Geometry check sheet. Reference: the model listing, model coordinates, mm. Face numbers are marked on the shaded views. A direction names the side the tool comes from. Coordinates: 2 decimals unless noted, no trailing zeros. Loops run counter-clockwise (first coordinate to the right, second up) from the corner with the lowest first, then second, coordinate; pieces in that order, holes last. Notation, with made-up numbers: (58, 70) -> (76, 70) arc R18 ccw to (76, 88) -> close; hole circle Ø11 at (66, -4.5). An arc over 180 degrees is marked (long way). Answer as a JSON object with one key per item and string values.
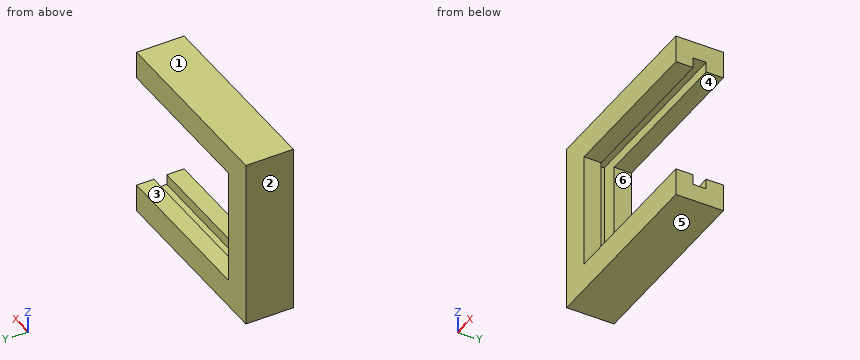
from build123d import *

# Parameters (mm, degrees)
SKETCH1_W           = 19.8
SKETCH1_H           = 5.5
SKETCH1_W_2         = 15.8
SKETCH1_H_2         = 1.5
BOSS_EXTRUDE1_DEPTH = 20.5
SKETCH2_W           = 18.5
SKETCH2_H           = 13.4
CUT_EXTRUDE1_DEPTH  = 6.5
SKETCH3_W           = 19.8
SKETCH3_H           = 5.5
BOSS_EXTRUDE2_DEPTH = 1.5


with BuildPart() as part:
    # Sketch1 → Boss-Extrude1 (new body)
    with BuildSketch(Plane(origin=(0, 0, 0), x_dir=(0, 0, -1), z_dir=(1, 0, 0))):
        with Locations((-4.788231672, 0.223036412)):
            Rectangle(SKETCH1_W, SKETCH1_H)
        with Locations((-4.788231672, 0.223036412)):
            Rectangle(SKETCH1_W_2, SKETCH1_H_2, mode=Mode.SUBTRACT)
    extrude(amount=BOSS_EXTRUDE1_DEPTH)

    # Sketch2 → Cut-Extrude1 (cut, through all)
    with BuildSketch(Plane(origin=(0, 2.973036412, 0), x_dir=(1, 0, 0), z_dir=(0, 1, 0))):
        with Locations((11.25, -4.788231672)):
            Rectangle(SKETCH2_W, SKETCH2_H)
    extrude(amount=-CUT_EXTRUDE1_DEPTH, mode=Mode.SUBTRACT)

    # Sketch3 → Boss-Extrude2 (add)
    with BuildSketch(Plane.ZY):
        with Locations((4.788231672, 0.223036412)):
            Rectangle(SKETCH3_W, SKETCH3_H)
    extrude(amount=BOSS_EXTRUDE2_DEPTH)


solid = part.part
1. Tool access check on the marked faces 5 and 6. Record the directions out of +Z, -Z, +X, -X, +Y, -Y that give a thin tool (end or side, any length) a straight path to the whole face; none if there is none.
Evaluation:
{"face 5": "-Z, +X, -X, +Y, -Y", "face 6": "+X, +Y, -Y"}
2. Mould release check, pull along Z, two halves, no side actions. Record for the marked faces 1, 2, 3 and 4: released by +Z, released by -Z, zero draft, split by the parting line, or undercut.
Evaluation:
{"face 1": "released by +Z", "face 2": "zero draft", "face 3": "undercut", "face 4": "undercut"}
3. Section check B-B, the plane z = 3.5. Record the boundary of the cut face in (x, y).
Evaluation:
{"outline": "(-1.5, -2.53) -> (2, -2.53) -> (2, -0.53) -> (0, -0.53) -> (0, 0.97) -> (2, 0.97) -> (2, 2.97) -> (-1.5, 2.97) -> close"}
4. Thickness scan on probe 1 along Z at (x, y) = (12.25, -0.9); probe 2 along Z at (x, y) = (11, 0.6); probe 3 along Y at (x, z) = (10, 12). Record the ranges inside material, lowest first. Write a range as from..to.
Evaluation:
{"probe 1": "z = -5.11..-1.91, 11.49..14.69", "probe 2": "z = -5.11..-3.11, 12.69..14.69", "probe 3": "y = -2.53..-0.53, 0.97..2.97"}
5. Depth check by flat-ended pin: P1, Ø1, axis at y = -1, z = 2.5, coming from the +X side. Enter the tip coordinate at first touch or a pass-through.
Evaluation:
{"P1": "stops at x = 2"}
6. Section check A-A, the plane x = 4.5. Record the boundary of the cut face in (y, z), then the cut area to 3 significant figures.
Evaluation:
{"outline": "(-2.53, -5.11) -> (2.97, -5.11) -> (2.97, -1.91) -> (0.97, -1.91) -> (0.97, -3.11) -> (-0.53, -3.11) -> (-0.53, -1.91) -> (-2.53, -1.91) -> close; (-2.53, 11.49) -> (-0.53, 11.49) -> (-0.53, 12.69) -> (0.97, 12.69) -> (0.97, 11.49) -> (2.97, 11.49) -> (2.97, 14.69) -> (-2.53, 14.69) -> close", "area": "31.6 mm^2"}
7. Section check C-C, the plane y = -1.1. Record the boundary of the cut face in (x, z), then the cut area to 3 significant figures.
Evaluation:
{"outline": "(-1.5, -5.11) -> (20.5, -5.11) -> (20.5, -1.91) -> (2, -1.91) -> (2, 11.49) -> (20.5, 11.49) -> (20.5, 14.69) -> (-1.5, 14.69) -> close", "area": "188 mm^2"}
